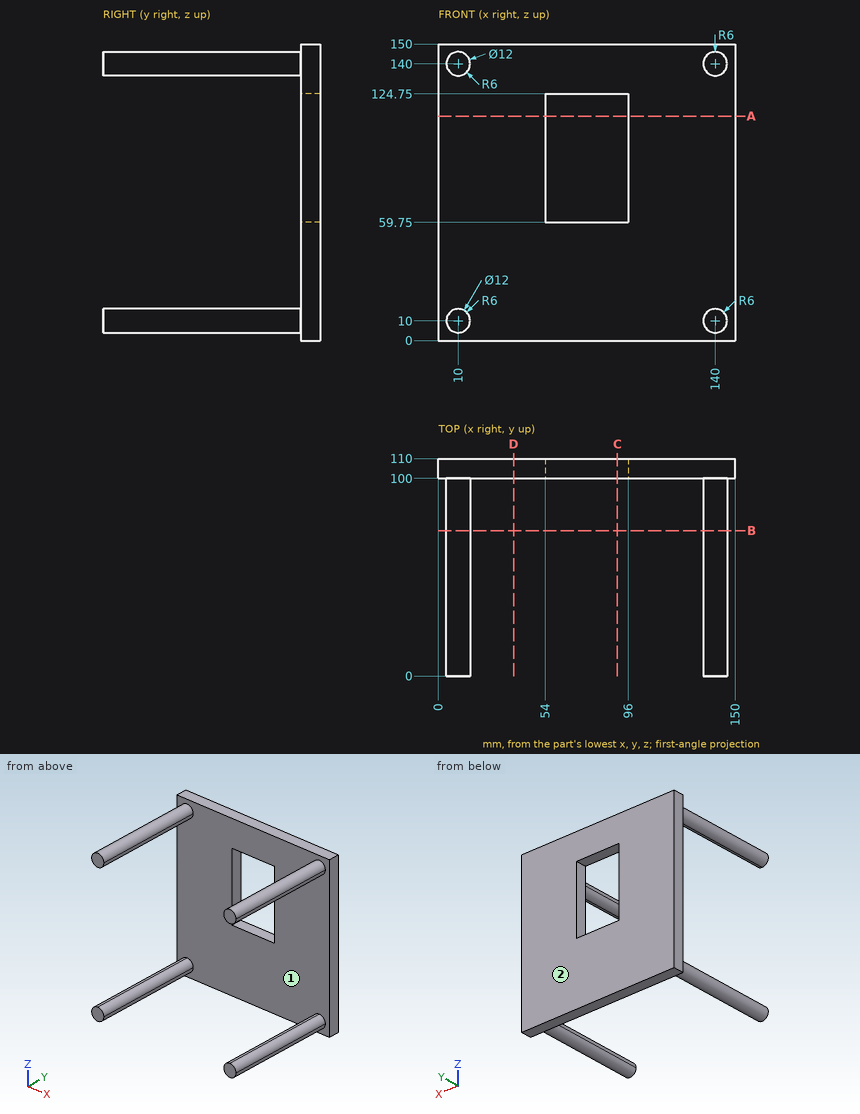
Answer from the drawing. Dimensions are ordinates in mm from the lowest x, y and z of the part. A direction names the side the tool comes from. Coordinates: 2 decimals unless noted, no trailing zeros. Write each loop counter-clockwise with the first axis right and the second up, starting at its lowest first coordinate (ties: lowest second). Pieces come first, ordered by that corner, then holes. Notation, with made-up numbers: M 26.25,-15.75 L 44.25,-15.75 A13 ccw 44.25,-2.75 Z; hole C 16.5,55 d7. An arc over 180 degrees is marked long. Use one line per item in the form item = value. Start each with the question number.
1. The part is cut by section C-C (x = 90.5). Give the vertices of the cut face in (y, z).
2. This flat-tipped pin is pushed along its axis until it touches: P1, Ø3, axis at x = 54, z = 127.5, coming from the -Y side. Where does it stop, or does it pass through?
3. Straight lines are drawn through the part: probe 1 along Z at (x, y) = (62.5, 102); probe 2 along Y at (x, z) = (54, 138.5); probe 3 along X at (y, z) = (51, 12.5). For each, find the intervals that lie inside material, in ascending order. Write a range as from..to.
4. The part is cut by section D-D (x = 38). Give the vertices of the cut face in (y, z).
5. A tool of negligible diameter and unlimited length cuts with its end or side. For the marked faces 1 and 2, from which of +Z, -Z, +X, -X, +Y, -Y can it reach the whole face along a straight path? Write none if from no direction.
6. The part is cut by section B-B (y = 73.5). Give the vertices of the cut face in (x, z), plus the area to 3 significant figures.
7. The part is cut by section A-A (z = 113.5). Give the vertices of the cut face in (x, y), plus the area to 3 significant figures.
Evaluation:
q1.outline = M 100,0 L 110,0 L 110,59.75 L 100,59.75 Z; M 100,124.75 L 110,124.75 L 110,150 L 100,150 Z
q2.P1 = 100
q3.probe_1 = 0..59.75, 124.75..150
q3.probe_2 = 100..110
q3.probe_3 = 4.55..15.45, 134.55..145.45
q4.outline = M 100,0 L 110,0 L 110,150 L 100,150 Z
q5.face_1 = -Y
q5.face_2 = +Z, -Z, +X, -X, +Y
q6.outline = C 10,10 d12; C 10,140 d12; C 140,10 d12; C 140,140 d12
q6.area = 452 mm^2
q7.outline = M 0,100 L 54,100 L 54,110 L 0,110 Z; M 96,100 L 150,100 L 150,110 L 96,110 Z
q7.area = 1,080 mm^2
